from build123d import *

# Parameters (mm, degrees)
SKETCH1_W           = 30
SKETCH1_H           = 18
BOSS_EXTRUDE1_DEPTH = 1
BOSS_EXTRUDE2_DEPTH = 18
FILLET1_R           = 2


with BuildPart() as part:
    # Sketch1 → Boss-Extrude1 (new body)
    with BuildSketch(Plane.XY):
        with Locations((-439.730210405, -52)):
            Rectangle(SKETCH1_W, SKETCH1_H)
    extrude(amount=BOSS_EXTRUDE1_DEPTH)

    # Sketch2 → Boss-Extrude2 (add)
    with BuildSketch(Plane(origin=(0, -43, 0), x_dir=(1, 0, 0), z_dir=(0, 1, 0))):
        with BuildLine():
            Line((-437.730210405, -1), (-441.730210405, -1))
            ThreePointArc((-441.730210405, -1), (-439.730210405, -3), (-437.730210405, -1))
        make_face()
    extrude(amount=-BOSS_EXTRUDE2_DEPTH)

    # Fillet1
    fillet1_edges = [part.edges().sort_by_distance(p)[0] for p in [
        (-454.730210405, -43, 0.5),
        (-424.730210405, -43, 0.5),
        (-454.730210405, -61, 0.5),
        (-424.730210405, -61, 0.5),
    ]]
    fillet(fillet1_edges, radius=FILLET1_R)


solid = part.part
Model file for the job. Use its own axes, mm. A direction names the side the tool comes from. Coordinates: 2 decimals unless noted, no trailing zeros. Loops run counter-clockwise (first coordinate to the right, second up) from the corner with the lowest first, then second, coordinate; pieces in that order, holes last. Notation, with made-up numbers: (64.5, 81.5) -> (71.5, 81.5) arc R13 ccw to (71.5, 93.5) -> close; hole circle Ø3 at (57, -7.75). An arc over 180 degrees is marked (long way). Use one line per item in the form item = value. Start each with the question number.
(1) Cut at C-C on z = 2.55. Give the cut face in (x, y), and give its area (3 significant figures).
(2) Tool access for faces 1 (the flat face through (-431, -52, 1)), 2 (the flat face through (-448, -52, 1)), 3 (the cylindrical face through (-439.8, -51.9, 3)): list every direction of +Z, -Z, +X, -X, +Y, -Y with a clear straight run to the whole face (end or side of a thin tool).
(3) Cut at A-A on y = -54.75. Give the cut face in (x, z).
(4) Flat gauge pins, fed straight in: pin 1 (1.5 mm diameter, centred on y = -54, z = 2.5, fed in from +X); pin 2 (2 mm diameter, centred on x = -444, y = -50.5, fed in from +Z). Where does each tip first touch, or does it go through?
(5) Cut at B-B on x = -450.75. Give the cut face in (y, z), and give its area (3 significant figures).
(6) Probe probe 1 along Z at (x, y) = (-448.25, -52.25); probe 2 along X at (y, z) = (-49, 1.05); probe 3 along X at (y, z) = (-52, 1.5). List the from-to ranges inside material, lowest first. Write a range as from..to.
Values:
q1.outline = (-440.99, -61) -> (-438.47, -61) -> (-438.47, -43) -> (-440.99, -43) -> close
q1.area = 45.5 mm2
q2.face_1 = +Z, +X, +Y, -Y
q2.face_2 = +Z, -X, +Y, -Y
q2.face_3 = +Z, +Y, -Y
q3.outline = (-454.73, 0) -> (-424.73, 0) -> (-424.73, 1) -> (-437.73, 1) arc R2 ccw to (-441.73, 1) -> (-454.73, 1) -> close
q4.pin_1 = -437.88
q4.pin_2 = 1
q5.outline = (-61, 0) -> (-43, 0) -> (-43, 1) -> (-61, 1) -> close
q5.area = 18.0 mm2
q6.probe_1 = 0..1
q6.probe_2 = -441.73..-437.73
q6.probe_3 = -441.67..-437.79
